Build history of the part. All positions in model axes, mm. Face numbers are marked on the shaded views. A direction names the side the tool comes from. Give positions to 0.01 mm unless a question says otherwise; leave off trailing zeros. Loops run counter-clockwise (first coordinate to the right, second up) from the corner with the lowest first, then second, coordinate; pieces in that order, holes last.
1) Band-saw the part on D-D on x = 1.55. State how many separate pieces and enclosed holes the cut face has, then the cut area to 3 significant figures.
2) Band-saw the part on B-B on x = 0. List the corners of the cut face in (y, z), then the cut area to 3 significant figures.
3) Flat gauge pins, fed straight in: P1, Ø3, axis at y = 10, z = 1, coming from the +X side; P2, Ø1.5, axis at x = 1.5, y = 3, coming from the +Z side; P3, Ø1, axis at x = 2, z = -2, coming from the -Y side. Where does each tip first touch, or does it go through?
4) Band-saw the part on A-A on z = 0. List the corners of the cut face in (x, y).
5) Two-plate mould, pull along Y, no slides. Class the marked faces 4, 5 and 6: +Y half, -Y half, draft (parallel to the pull), parting line (faces both ways), or undercut.
6) Band-saw the part on C-C on y = 9. List the corners of the cut face in (x, z).
7) 3-axis set-ups, long thin cutter, end or side, ignore diameter. For the marked faces 1, 2 and 3: which of +Z, -Z, +X, -X, +Y, -Y reach the whole face in a straight line?
8) Wall check: line 1 (Z direction, x = 0, y = 4.25); line 2 (Z direction, x = 0, y = 6.25). Give the ranges that are in metal, low to high.
Autodesk Inventor part; units mm, degrees
ref_plane "YZ Plane" through (0, 0, 0) normal (1, 0, 0) x (0, 1, 0)
ref_plane "XZ Plane" through (0, 0, 0) normal (0, 1, 0) x (-1, 0, 0)
ref_plane "XY Plane" through (0, 0, 0) normal (0, 0, 1) x (1, 0, 0)
sketch "Sketch1" plane through (0, 0, 0) normal (0, 0, 1) x (1, 0, 0)
  line L0 (-2, 0) -> (-2, 5)
  line L1 (-2, 5) -> (-3, 6)
  line L2 (-3, 6) -> (-3, 7)
  line L3 (-3, 7) -> (-1.4, 8)
  line L4 (-0.9, 15) -> (-0.9, 0)
  line L5 (-0.9, 0) -> (-2, 0)
  line L6 (0, 18) -> (0, -3) construction
  line L7 (-3.6, 0) -> (0.6, 0) construction
  line L8 (-0.9, 15) -> (-1.2, 14.7)
  line L9 (-1.2, 14.7) -> (-1.2, 14.4)
  line L10 (-1.2, 14.4) -> (-1.8, 12.8)
  line L11 (-1.8, 12.8) -> (-1.4, 11.2)
  line L12 (-1.4, 11.2) -> (-1.8, 9.6)
  line L13 (-1.8, 9.6) -> (-1.4, 8)
  point P0 (0, 0)
  point P1 (-2, 2.5)
  dimension "d0" = 15
  dimension "d4" = 1
  dimension "d5" = 0.9
  dimension "d6" = 1.8
  dimension "d9" = 5
  dimension "d10" = 1
  dimension "d11" = 1
  dimension "d12" = 2.5
  dimension "d14" = 2
  dimension "d15" = 1.2
  dimension "d16" = 1.8
  dimension "d17" = 3
  dimension "d18" = 45
  dimension "d19" = 0.3
  dimension "d20" = 1.4
  dimension "d21" = 1.4
  dimension "d22" = 1.6
  dimension "d23" = 1.6
  dimension "d24" = 1.6
revolve "Revolution1" add sketch "Sketch1" angle 360 about axis through (0, 0, 0) along (0, -1, 0)
properties part number "Thread to Barbed 3-32 inch and 10-32 hole"
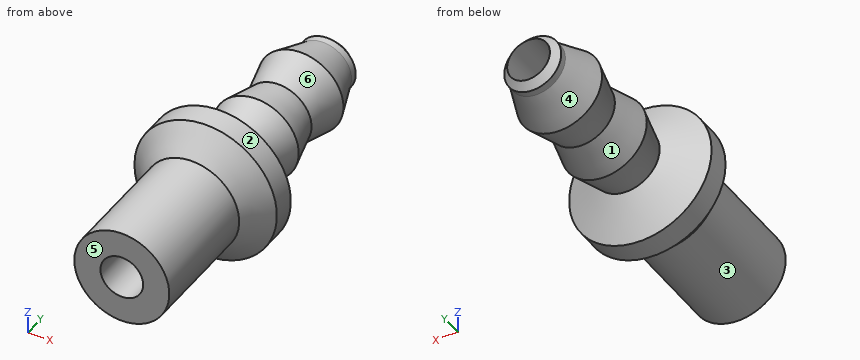
Findings below:
1. separate pieces: 3
1. enclosed holes: 0
1. area: 29.0 mm2
2. outline: (0, -2) - (5, -2) - (6, -3) - (7, -3) - (8, -1.4) - (9.6, -1.8) - (11.2, -1.4) - (12.8, -1.8) - (14.4, -1.2) - (14.7, -1.2) - (15, -0.9) - (0, -0.9) - close; (0, 0.9) - (15, 0.9) - (14.7, 1.2) - (14.4, 1.2) - (12.8, 1.8) - (11.2, 1.4) - (9.6, 1.8) - (8, 1.4) - (7, 3) - (6, 3) - (5, 2) - (0, 2) - close
2. area: 29.9 mm2
3. P1: stops at x = 1.8
3. P2: stops at z = 1.85
3. P3: stops at y = 5.33
4. outline: (-3, 6) - (-2, 5) - (-2, 0) - (-0.9, 0) - (-0.9, 15) - (-1.2, 14.7) - (-1.2, 14.4) - (-1.8, 12.8) - (-1.4, 11.2) - (-1.8, 9.6) - (-1.4, 8) - (-3, 7) - close; (0.9, 0) - (2, 0) - (2, 5) - (3, 6) - (3, 7) - (1.4, 8) - (1.8, 9.6) - (1.4, 11.2) - (1.8, 12.8) - (1.2, 14.4) - (1.2, 14.7) - (0.9, 15) - close
5. face 4: +Y half
5. face 5: -Y half
5. face 6: undercut
6. outline: circle Ø3.3 at (0, 0); hole circle Ø1.8 at (0, 0)
7. face 1: none
7. face 2: +Y, -Y
7. face 3: -Y
8. line 1: z = -2 to -0.9, 0.9 to 2
8. line 2: z = -3 to -0.9, 0.9 to 3
